Model file for the job. Use its own axes, mm. A direction names the side the tool comes from. Round coordinates to 2 decimals unless told otherwise and drop trailing zeros. Loops run counter-clockwise (first coordinate to the right, second up) from the corner with the lowest first, then second, coordinate; pieces in that order, holes last. Notation, with made-up numbers: M -34.5,48.25 L -17.5,48.25 A17 cw -17.5,76.25 Z; hole C 63,80.5 d4. An arc over 180 degrees is marked long. Answer in a Markdown table with one row per item.
from build123d import *

# Parameters (mm, degrees)
BOSS_EXTRUDE1_DEPTH = 5


with BuildPart() as part:
    # Sketch1 → Boss-Extrude1 (new body)
    with BuildSketch(Plane.XY):
        Polygon((-10.211091397, -1.328977692), (-15.204731397, -16.328947692), (-15.204731397, -22.678947692), (-8.854731397, -22.678947692), (-8.854731397, -16.328947692), (-2.405671397, -16.328947692), (-2.405671397, -11.329465692), (-4.706911397, -11.329465692), (-4.706911397, -7.328965692), (-2.405671397, -7.328965692), (-2.405671397, -2.629965692), (1.988528603, -2.629965692), (1.988528603, -7.328965692), (4.292308603, -7.328965692), (4.292308603, -11.329465692), (1.988528603, -11.329465692), (1.988528603, -16.328947692), (8.442668603, -16.328947692), (8.442668603, -22.678947692), (14.792668603, -22.678947692), (14.792668603, -16.328947692), (9.788868603, -1.328977692), (9.788868603, 9.134552308), (7.292048603, 9.134552308), (7.292048603, 15.485060308), (9.517088603, 15.485060308), (9.382468603, 16.046400308), (8.719528603, 17.669460308), (7.459688603, 19.584620308), (5.795988603, 21.164500308), (4.317708603, 22.106840308), (3.789388603, 22.335440308), (-4.209071397, 22.335440308), (-4.737391397, 22.106840308), (-6.215671397, 21.167040308), (-7.881911397, 19.584620308), (-9.141751397, 17.669460308), (-9.804691397, 16.048940308), (-9.939311397, 15.485060308), (-7.709191397, 15.485060308), (-7.709191397, 9.134552308), (-10.211091397, 9.134552308), align=None)
        Polygon((1.988528603, 12.309552308), (1.988528603, 12.524182308), (1.815808603, 13.166548308), (1.343368603, 13.866572308), (0.644868603, 14.337996308), (0.002248603, 14.509954308), (-0.211111397, 14.509954308), (-0.427011397, 14.509954308), (-1.069631397, 14.337996308), (-1.768131397, 13.866572308), (-2.240571397, 13.166548308), (-2.413291397, 12.524182308), (-2.413291397, 12.309552308), (-2.413291397, 12.095684308), (-2.240571397, 11.453572308), (-1.768131397, 10.755072308), (-1.069631397, 10.283648308), (-0.427011397, 10.110166308), (-0.211111397, 10.110166308), (0.002248603, 10.110166308), (0.644868603, 10.283648308), (1.343368603, 10.755072308), (1.815808603, 11.453572308), (1.988528603, 12.095684308), align=None, mode=Mode.SUBTRACT)
    extrude(amount=BOSS_EXTRUDE1_DEPTH)


solid = part.part
1. Saw through at C-C (y = 8.5). Write the cut outline in (x, z).
Verdict:
| item | result |
|---|---|
| outline | M -10.21,0 L 9.79,0 L 9.79,5 L -10.21,5 Z |
2. Saw through at B-B (x = -3). Write the cut outline in (y, z), and give its area (3 significant figures).
Verdict:
| item | result |
|---|---|
| outline | M -16.33,0 L -11.33,0 L -11.33,5 L -16.33,5 Z; M -7.33,0 L 22.34,0 L 22.34,5 L -7.33,5 Z |
| area | 173 mm² |
3. Pin check, flat tips, straight feed: pin 1 (2.5 mm diameter, centred on y = 11.5, z = 3, fed in from +X); pin 2 (3 mm diameter, centred on x = 3.5, y = 14.5, fed in from -Z); pin 3 (2.5 mm diameter, centred on y = 4.5, z = 1.5, fed in from -X); pin 4 (1 mm diameter, centred on x = 5, z = 1.5, fed in from +Y). Stop position of each tip, or through.
Verdict:
| item | result |
|---|---|
| pin 1 | stops at x = 7.29 |
| pin 2 | stops at z = 0 |
| pin 3 | stops at x = -10.21 |
| pin 4 | stops at y = 21.99 |
4. Wall check: probe 1 along X at (y, z) = (-19.5, 3.5); probe 2 along X at (y, z) = (5, 2.4); probe 3 along X at (y, z) = (10, 3.4). Give the ranges that are in metal, low to high.
Verdict:
| item | result |
|---|---|
| probe 1 | x = -15.2 to -8.85, 8.44 to 14.79 |
| probe 2 | x = -10.21 to 9.79 |
| probe 3 | x = -7.71 to 7.29 |
5. Tool access for faces 1 (the flat face through (5.067, 21.629, 2.465)), 2 (the flat face through (-2.406, -5, 2)), 3 (the flat face through (8, 15.485, 2)), 4 (the flat face through (-7.709, 12, 2)), 5 (the flat face through (-4, -11.329, 2)): list every direction of +Z, -Z, +X, -X, +Y, -Y with a clear straight run to the whole face (end or side of a thin tool).
Verdict:
| item | result |
|---|---|
| face 1 | +Z, -Z, +X, +Y |
| face 2 | +Z, -Z, -Y |
| face 3 | +Z, -Z, +X |
| face 4 | +Z, -Z, -X |
| face 5 | +Z, -Z |
6. Saw through at A-A (y = -17). Write the cut outline in (x, z), and give its area (3 significant figures).
Verdict:
| item | result |
|---|---|
| outline | M -15.2,0 L -8.85,0 L -8.85,5 L -15.2,5 Z; M 8.44,0 L 14.79,0 L 14.79,5 L 8.44,5 Z |
| area | 63.5 mm² |
7. Mould opens along Y. For faces 6 (the flat face through (7.292, 12, 2)), 7 (the flat face through (-9, 9.135, 2)), 8 (the flat face through (-12.67, -8.72, 2.46)), 9 (the flat face through (-12, -22.679, 2)) say: +Y half, -Y half, draft (parallel to the pull), parting line (faces both ways), or undercut.
Verdict:
| item | result |
|---|---|
| face 6 | undercut |
| face 7 | undercut |
| face 8 | +Y half |
| face 9 | -Y half |
8. Saw through at D-D (x = 6.75). Write the cut outline in (y, z), and give its area (3 significant figures).
Verdict:
| item | result |
|---|---|
| outline | M -16.33,0 L 20.26,0 L 20.26,5 L -16.33,5 Z |
| area | 183 mm² |
